Build history of the part. All positions in model axes, mm. Face numbers are marked on the shaded views. A direction names the side the tool comes from. Give positions to 0.01 mm unless a question says otherwise; leave off trailing zeros. Loops run counter-clockwise (first coordinate to the right, second up) from the corner with the lowest first, then second, coordinate; pieces in that order, holes last.
1) Band-saw the part on B-B on y = 0. List the corners of the cut face in (x, z), then the cut area to 3 significant figures.
2) Band-saw the part on C-C on z = 3.8. List the corners of the cut face in (x, y), then the cut area to 3 significant figures.
3) Flat gauge pins, fed straight in: P1, Ø0.7, axis at x = 3.5, y = 0, coming from the -Z side; P2, Ø6, axis at x = 0, y = -4, coming from the +Z side; P3, Ø1, axis at y = -2.5, z = 4, coming from the -X side. Where does each tip first touch, or does it go through?
4) Band-saw the part on D-D on x = 0. List the corners of the cut face in (y, z).
5) Band-saw the part on A-A on z = 0.6. List the corners of the cut face in (x, y).
6) 3-axis set-ups, long thin cutter, end or side, ignore diameter. For the marked faces 1, 2 and 3: which of +Z, -Z, +X, -X, +Y, -Y reach the whole face in a straight line?
7) Wall check: line 1 (Y direction, x = 4, z = 2.5); line 2 (X direction, y = -7.25, z = 1.25); line 3 (Y direction, x = 3.75, z = 0.6). Give the ranges that are in metal, low to high.
8) Two-plate mould, pull along Y, no slides. Class the marked faces 4, 5, 6 and 7: +Y half, -Y half, draft (parallel to the pull), parting line (faces both ways), or undercut.
Autodesk Inventor part; units mm, degrees
ref_plane "YZ Plane" through (0, 0, 0) normal (1, 0, 0) x (0, 1, 0)
ref_plane "XZ Plane" through (0, 0, 0) normal (0, 1, 0) x (-1, 0, 0)
ref_plane "XY Plane" through (0, 0, 0) normal (0, 0, 1) x (1, 0, 0)
sketch "Sketch1" plane through (0, 0, 0) normal (0, 0, 1) x (1, 0, 0)
  line L0 (-8, 12) -> (8, 12)
  line L1 (8, 12) -> (8, -12)
  line L2 (8, -12) -> (-8, -12)
  line L3 (-8, -12) -> (-8, 12)
  point P0 (0, 0)
  dimension "d0" = 16
  dimension "d1" = 24
  dimension "d2" = 8
  dimension "d3" = 12
extrude "Extrusion1" add sketch "Sketch1" along normal blind 3.2
shell "Shell1" thickness 1.5 removed faces 1 at (2.6667, 4, 0)
sketch "Sketch2" plane through (0, 0, 3.2) normal (0, 0, 1) x (1, 0, 0)
  circle A0 centre (4, -8) radius 2.5
  line L0 (8, 12) -> (8, -12)
  line L1 (8, -12) -> (-8, -12)
  dimension "d7" = 5
  dimension "d10" = 4
  dimension "d11" = 4
extrude "Extrusion2" add sketch "Sketch2" along normal blind 1.6
sketch "Sketch3" plane through (6.5, -10.5, 1.7) normal (0, 0, -1) x (-1, 0, 0)
  circle A0 centre (2.5, 2.5) radius 2.5
  circle A1 centre (2.5, 2.5) radius 1.2
  point P0 (6.5, 10.5)
  dimension "d18" = 2.4
extrude "Extrusion3" cut sketch "Sketch3" against normal blind 1.6 contours A1
pattern_linear "Rectangular Pattern1" count 3 spacing 8 along (0, 1, 0) count 2 spacing 8 along (-1, 0, 0) of "Extrusion2", "Extrusion3"
sketch "Sketch4" plane through (6.5, -10.5, 1.7) normal (0, 0, -1) x (-1, 0, 0)
  circle A0 centre (2.5, 10.5) radius 1.2
  circle A1 centre (2.5, 2.5) radius 1.2
  line L0 (0, 21) -> (0, 0)
  line L1 (0, 0) -> (13, 0)
  circle A2 centre (6.5, 6.5) radius 3.15
  circle A3 centre (6.5, 6.5) radius 2.5
  point P0 (6.5, 10.5)
  dimension "d21" = 6.5
  dimension "d22" = 6.5
  dimension "d23" = 10.5
  dimension "d24" = 2.5
  dimension "d25" = 5
  dimension "d26" = 6.3
extrude "Extrusion4" add sketch "Sketch4" along normal up to surface (1.7 mm away) contours A2
pattern_linear "Rectangular Pattern2" count 2 spacing 8 along (0, 1, 0) of "Extrusion4"
equation "\"d0\" = 0.8 * WIDTH"
equation "\"d1\" = 0.8 * LENGTH"
equation "\"d4\" = HEIGHT"
equation "\"d21\" = 0.5 * d23 + 0.5 * d24"
equation "\"d22\" = d21"
equation "\"WIDTH\" = 2"
equation "\"HEIGHT\" = 3.2"
properties part number "3021" material "Steel"
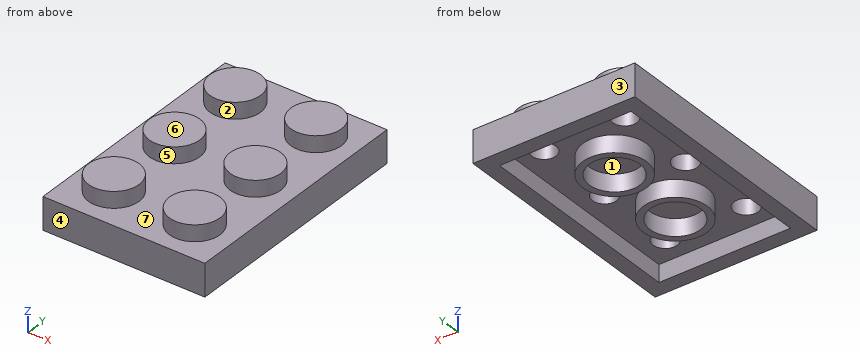
Findings below:
1. outline: (-8, 0) - (-6.5, 0) - (-6.5, 1.7) - (-5.2, 1.7) - (-5.2, 3.3) - (-2.8, 3.3) - (-2.8, 1.7) - (2.8, 1.7) - (2.8, 3.3) - (5.2, 3.3) - (5.2, 1.7) - (6.5, 1.7) - (6.5, 0) - (8, 0) - (8, 3.2) - (6.5, 3.2) - (6.5, 4.8) - (1.5, 4.8) - (1.5, 3.2) - (-1.5, 3.2) - (-1.5, 4.8) - (-6.5, 4.8) - (-6.5, 3.2) - (-8, 3.2) - close
1. area: 37.4 mm2
2. outline: circle Ø5 at (-4, -8); circle Ø5 at (-4, 0); circle Ø5 at (-4, 8); circle Ø5 at (4, -8); circle Ø5 at (4, 0); circle Ø5 at (4, 8)
2. area: 118 mm2
3. P1: stops at z = 3.3
3. P2: stops at z = 3.2
3. P3: stops at x = -5.5
4. outline: (-12, 0) - (-10.5, 0) - (-10.5, 1.7) - (-7.15, 1.7) - (-7.15, 0) - (-6.5, 0) - (-6.5, 1.7) - (-1.5, 1.7) - (-1.5, 0) - (-0.85, 0) - (-0.85, 1.7) - (0.85, 1.7) - (0.85, 0) - (1.5, 0) - (1.5, 1.7) - (6.5, 1.7) - (6.5, 0) - (7.15, 0) - (7.15, 1.7) - (10.5, 1.7) - (10.5, 0) - (12, 0) - (12, 3.2) - (-12, 3.2) - close
5. outline: (-8, -12) - (8, -12) - (8, 12) - (-8, 12) - close; circle Ø6.3 at (0, -4); circle Ø6.3 at (0, 4); hole (-6.5, -10.5) - (6.5, -10.5) - (6.5, 10.5) - (-6.5, 10.5) - close; hole circle Ø5 at (0, -4); hole circle Ø5 at (0, 4)
6. face 1: -Z
6. face 2: +Z
6. face 3: +Z, -Z, +X, -X, +Y
7. line 1: y = -12 to -9.2, -6.8 to -1.2, 1.2 to 6.8, 9.2 to 12
7. line 2: x = -8 to -6.5, 6.5 to 8
7. line 3: y = -12 to -10.5, 10.5 to 12
8. face 4: -Y half
8. face 5: undercut
8. face 6: draft
8. face 7: undercut
